```python
from build123d import *

# Parameters (mm, degrees)
SKETCH1_R             = 4
BOSS_EXTRUDE1_DEPTH   = 2
CIRPATTERN1_OUTLINE_R = 4
CIRPATTERN1_DEPTH     = 2


# Read off the part's stored shape, not the designer's step: CirPattern1
with BuildPart() as part:
    # Sketch1 → Boss-Extrude1 (new body)
    with BuildSketch(Plane.XY):
        with BuildLine():
            Line((0, 1250), (0, 175))
            ThreePointArc((0, 175), (102.995768235, 141.480994221), (166.536499319, 53.764248293))
            Line((166.536499319, 53.764248293), (1188.922508468, 385.957599819))
            ThreePointArc((1188.922508468, 385.957599819), (734.864953657, 1011.17431726), (0, 1250))
        make_face()
        with Locations((206.086847975, 77.543569361)):
            Circle(SKETCH1_R, mode=Mode.SUBTRACT)
        with Locations((529.567521621, 182.234800025)):
            Circle(SKETCH1_R, mode=Mode.SUBTRACT)
        with Locations((852.926737161, 287.300578112)):
            Circle(SKETCH1_R, mode=Mode.SUBTRACT)
        with Locations((10, 219.959676764)):
            Circle(SKETCH1_R, mode=Mode.SUBTRACT)
        with Locations((10, 559.959676764)):
            Circle(SKETCH1_R, mode=Mode.SUBTRACT)
        with Locations((10, 899.959676764)):
            Circle(SKETCH1_R, mode=Mode.SUBTRACT)
        with Locations((10, 1239.959676764)):
            Circle(SKETCH1_R, mode=Mode.SUBTRACT)
        with Locations((1176.285952701, 392.3663562)):
            Circle(SKETCH1_R, mode=Mode.SUBTRACT)
    extrude(amount=BOSS_EXTRUDE1_DEPTH)

    # CirPattern1 outline → CirPattern1 (cut)
    with BuildSketch(Plane.XY):
        with Locations((248.343744291, 1214.876695254)):
            Circle(CIRPATTERN1_OUTLINE_R)
        with Locations((554.314862591, 1109.204684948)):
            Circle(CIRPATTERN1_OUTLINE_R)
        with Locations((822.510339054, 927.94220841)):
            Circle(CIRPATTERN1_OUTLINE_R)
        with Locations((1034.653095173, 683.442003866)):
            Circle(CIRPATTERN1_OUTLINE_R)
    extrude(amount=CIRPATTERN1_DEPTH, mode=Mode.SUBTRACT)


solid = part.part
```
Here's how the part is built. I have some questions about the finished solid (model axes, mm). Round coordinates to 2 decimals unless told otherwise and drop trailing zeros. Loops run counter-clockwise (first coordinate to the right, second up) from the corner with the lowest first, then second, coordinate; pieces in that order, holes last. Notation, with made-up numbers: (56, 49) -> (86, 49) arc R20 ccw to (86, 56) -> close; hole circle Ø8 at (-30.75, -24). An arc over 180 degrees is marked (long way). Answer as CSV lines item,"result". Start each with the question number.
1. Imagine slicing it at C-C on x = 466. Write out the boundary of the cut face in (y, z), plus the area to 3 significant figures.
2. Imagine slicing it at B-B on y = 830. Write out the boundary of the cut face in (x, z).
3. I'm going to push a flat-ended pin straight in: P1, Ø13, axis at x = 1034.65, y = 683.44, coming from the -Z side. Where does the tip first touch, or does it pass through?
4. Imagine slicing it at A-A on z = 1.1. State how many separate pieces and enclosed holes the cut face has, plus the area to 3 significant figures.
5. I need wall thicknesses on probe 1 along Y at (x, z) = (10, 0.6); probe 2 along X at (y, z) = (1111, 1.6); probe 3 along X at (y, z) = (984.5, 0.45). Which ranges of each line are inside material? Lowest first, please. Write a range as from..to.
Solution:
1,outline,"(151.07, 0) -> (1159.89, 0) -> (1159.89, 2) -> (151.07, 2) -> close"
1,area,"2,020 mm²"
2,outline,"(0, 0) -> (934.67, 0) -> (934.67, 2) -> (0, 2) -> close"
3,P1,"z = 0"
4,separate pieces,"1"
4,enclosed holes,"12"
4,area,"962,000 mm²"
5,probe 1,"174.71..215.96, 223.96..555.96, 563.96..895.96, 903.96..1235.96, 1243.96..1249.96"
5,probe 2,"0..550.74, 557.89..572.87"
5,probe 3,"0..770.23"
